from build123d import *

# Parameters (mm, degrees)
BOSS_EXTRUDE1_DEPTH = 22.5
SKETCH2_W           = 3.36
SKETCH2_H           = 28
CUT_EXTRUDE1_DEPTH  = 54.046862301
SKETCH3_W           = 7.36
SKETCH3_H           = 13
CUT_EXTRUDE2_DEPTH  = 54.046862301
SKETCH4_R           = 4.69
SKETCH4_R_2         = 3.835
CUT_EXTRUDE3_DEPTH  = 10
SKETCH6_R           = 4.775
CUT_EXTRUDE5_DEPTH  = 2
RIB2_REACH          = 55.047
SKETCH7_WALL_W      = 127.943157844
SKETCH7_WALL_H      = 1.5
RIB3_START          = -1.5
RIB3_DEPTH          = 1.5
RIB4_REACH          = 37.989
SKETCH9_WALL_W      = 93.8277522
SKETCH9_WALL_H      = 2


# Read off the part's stored shape, not the designer's step: Rib3
with BuildPart() as part:
    # Sketch1 → Boss-Extrude1 (new, symmetric)
    with BuildSketch(Plane(origin=(0, 0, 0), x_dir=(0, 0, -1), z_dir=(1, 0, 0))):
        Polygon((0, -13), (0, 17), (-7.36, 17), (-7.36, 4), (-22.36, 4), (-22.36, 0), (-7.36, 0), (-7.36, -13), align=None)
    extrude(amount=BOSS_EXTRUDE1_DEPTH, both=True)

    # Sketch2 → Cut-Extrude1 (cut, through all)
    with BuildSketch(Plane(origin=(22.5, 0, 0), x_dir=(0, 0, -1), z_dir=(1, 0, 0))):
        with Locations((-3.68, 1)):
            Rectangle(SKETCH2_W, SKETCH2_H)
    extrude(amount=-CUT_EXTRUDE1_DEPTH, mode=Mode.SUBTRACT)

    # Sketch3 → Cut-Extrude2 (cut, through all)
    with BuildSketch(Plane(origin=(22.5, 0, 0), x_dir=(0, 0, -1), z_dir=(1, 0, 0))):
        with Locations((-3.68, -6.5)):
            Rectangle(SKETCH3_W, SKETCH3_H)
    extrude(amount=-CUT_EXTRUDE2_DEPTH, mode=Mode.SUBTRACT)

    # Sketch4 → Cut-Extrude3 (cut)
    with BuildSketch(Plane(origin=(0, 0, 0), x_dir=(-1, 0, 0), z_dir=(0, -1, 0))):
        with Locations(Location((-12.5, -14.36, 0), (0, 0, 90))):
            Circle(SKETCH4_R)
        with Locations(Location((12.5, -14.36, 0), (0, 0, 90))):
            Circle(SKETCH4_R_2)
    extrude(amount=-CUT_EXTRUDE3_DEPTH, mode=Mode.SUBTRACT)

    # Sketch6 → Cut-Extrude5 (cut)
    with BuildSketch(Plane(origin=(0, 0, 0), x_dir=(-1, 0, 0), z_dir=(0, -1, 0))):
        with Locations(Location((-12.5, -14.36, 0), (0, 0, 90))):
            Circle(SKETCH6_R)
    extrude(amount=-CUT_EXTRUDE5_DEPTH, mode=Mode.SUBTRACT)

    # Sketch7 wall → Rib2 (add, up to next)
    with BuildSketch(Plane(origin=(-22.5, 10.5, 14.86), x_dir=(0, 0.654930538418, -0.75568908279), z_dir=(0, -0.75568908279, -0.654930538418)), mode=Mode.PRIVATE) as rib2_sk1:
        with Locations((0, 0.75)):
            Rectangle(SKETCH7_WALL_W, SKETCH7_WALL_H)
    rib2_tool1 = extrude(rib2_sk1.sketch, amount=RIB2_REACH, mode=Mode.PRIVATE) - part.part
    add(rib2_tool1.solids().sort_by_distance((-22.5, 10.5, 14.86))[0])

    # Rib3 outline → Rib3 (add)
    with BuildSketch(Plane(origin=(22.5, 0, 0), x_dir=(0, 0, -1), z_dir=(1, 0, 0)).offset(RIB3_START)):
        Polygon((-7.36, 17), (-22.36, 4), (-7.36, 4), align=None)
    extrude(amount=RIB3_DEPTH)

    # Sketch9 wall → Rib4 (add, up to next)
    with BuildSketch(Plane(origin=(0, 10.5, 14.86), x_dir=(0, 0.654930538418, -0.75568908279), z_dir=(0, 0.75568908279, 0.654930538418)), mode=Mode.PRIVATE) as rib4_sk1:
        Rectangle(SKETCH9_WALL_W, SKETCH9_WALL_H)
    rib4_tool1 = extrude(rib4_sk1.sketch, amount=-RIB4_REACH, mode=Mode.PRIVATE) - part.part
    add(rib4_tool1.solids().sort_by_distance((0, 10.5, 14.86))[0])


solid = part.part
Read the model definition and answer for the solid it produces. Units are mm, in the model's axes. A direction names the side the tool comes from. Coordinates: 2 decimals unless noted, no trailing zeros. Write each loop counter-clockwise with the first axis right and the second up, starting at its lowest first coordinate (ties: lowest second). Pieces come first, ordered by that corner, then holes. Notation, with made-up numbers: M 47,18.25 L 71,18.25 A36 cw 71,54.25 Z; hole C -30.5,-12.5 d9. An arc over 180 degrees is marked long. Use a Markdown table: item, result.
Q1. Each of these flat-tipped pins is pushed along its axis until it touches: pin 1 Ø1 at (x, z) = (15.5, 9) entering from +Y; pin 2 Ø2.5 at (x, z) = (-9, 3.5) entering from -Y; pin 3 Ø4.5 at (x, y) = (-9, 9) entering from +Z. Where does it stop, or does it pass through?
Answer block:
| item | result |
|---|---|
| pin 1 | stops at y = 4 |
| pin 2 | stops at y = 15 |
| pin 3 | stops at z = 7.36 |
Q2. Determine the mould class of faces 1 (the face through (1, 8, 13)), 2 (the face through (0, 7, 5.36)), 3 (the face through (-22.5, 8, 11)), 4 (the face through (-1, 8, 13)) for opening direction X: released by +X, released by -X, zero draft, split by the parting line, or undercut.
Answer block:
| item | result |
|---|---|
| face 1 | undercut |
| face 2 | zero draft |
| face 3 | released by -X |
| face 4 | undercut |
Q3. Which of the six approach directions +Z, -Z, +X, -X, +Y, -Y give full straight-line access (tool end or side, diameter ignored) to faces 5 (the face through (11, 11, 7.36)), 6 (the face through (22.5, 7, 11)), 7 (the face through (0, 15, 4)), 8 (the face through (10.67, 0.99, 9.95))?
Answer block:
| item | result |
|---|---|
| face 5 | +Z, +Y |
| face 6 | +Z, -Z, +X, +Y, -Y |
| face 7 | +X, -X, -Y |
| face 8 | -Y |
Q4. Straight lines are drawn through the part: L1, parallel to X at y = 9.75, z = 9.75; L2, parallel to X at y = 1.65, z = 14.36 (3 decimals); L3, parallel to Z at x = 3, y = 7.5. For each, find the intervals that lie inside material, in ascending order. Write a range as [from, to].
Answer block:
| item | result |
|---|---|
| L1 | x = [-22.5, -21], [-1, 1], [21, 22.5] |
| L2 | x = [-22.5, -16.335], [-8.665, 7.725], [17.275, 22.5] |
| L3 | z = [0, 2], [5.36, 7.36] |
Q5. The part is cut by section A-A, the plane x = -12.5. Write down the section's boundary in (y, z) (3 decimals).
Answer block:
| item | result |
|---|---|
| outline | M 0,0 L 17,0 L 17,7.36 L 4,7.36 L 4,10.525 L 0,10.525 L 0,5.36 L 15,5.36 L 15,2 L 0,2 Z; M 0,18.195 L 4,18.195 L 4,22.36 L 0,22.36 Z |
Q6. The part is cut by section B-B, the plane y = 11. Write down the section's boundary in (x, z).
Answer block:
| item | result |
|---|---|
| outline | M -22.5,0 L 22.5,0 L 22.5,2 L -22.5,2 Z; M -22.5,5.36 L 22.5,5.36 L 22.5,14.28 L 21,14.28 L 21,7.36 L 1,7.36 L 1,14.28 L -1,14.28 L -1,7.36 L -21,7.36 L -21,14.28 L -22.5,14.28 Z |
Q7. The part is cut by section C-C, the plane z = 16.5. Write down the section's boundary in (x, y).
Answer block:
| item | result |
|---|---|
| outline | M -22.5,0 L -15.68,0 L -15.68,4 L -21,4 L -21,9.08 L -22.5,9.08 Z; M -9.32,0 L 8.23,0 L 8.23,2 L 8.33,2 L 8.33,4 L 1,4 L 1,9.08 L -1,9.08 L -1,4 L -9.32,4 Z; M 16.67,2 L 16.77,2 L 16.77,0 L 22.5,0 L 22.5,9.08 L 21,9.08 L 21,4 L 16.67,4 Z |
Q8. The part is cut by section D-D, the plane x = -17.5. Write down the section's boundary in (y, z), then the cut area to 3 significant figures.
Answer block:
| item | result |
|---|---|
| outline | M 0,0 L 17,0 L 17,7.36 L 4,7.36 L 4,22.36 L 0,22.36 L 0,5.36 L 15,5.36 L 15,2 L 0,2 Z |
| area | 135 mm2 |
